Geometry: final body of the model. Coordinates: model frame, mm. Round coordinates to 2 decimals unless told otherwise and drop trailing zeros. Answer in a Markdown table with one row per item.
```python
from build123d import *

# Parameters (mm, degrees)
SKETCH1_R           = 2.25
BOSS_EXTRUDE1_DEPTH = 28


with BuildPart() as part:
    # Sketch1 → Boss-Extrude1 (new body)
    with BuildSketch(Plane(origin=(0, 0, 0), x_dir=(0, 0, -1), z_dir=(1, 0, 0))):
        with BuildLine():
            Line((-150, 25), (150, 25))
            add(Edge.make_bspline(
                [(150, 25), (230, 0), (150, -25)],
                knots=[0, 0, 0, 1, 1, 1], degree=2))
            Line((150, -25), (-150, -25))
            add(Edge.make_bspline(
                [(-150, 25), (-230, 0), (-150, -25)],
                knots=[0, 0, 0, 1, 1, 1], degree=2))
        make_face()
        with Locations((-175, 0)):
            Circle(SKETCH1_R, mode=Mode.SUBTRACT)
        with Locations((175, 0)):
            Circle(SKETCH1_R, mode=Mode.SUBTRACT)
    extrude(amount=BOSS_EXTRUDE1_DEPTH)


solid = part.part
```
Item 1: Ray query, L1, parallel to Y at x = 9.25, z = 175; L2, parallel to Y at x = 21, z = 165; L3, parallel to Z at x = 25.75, y = -19.5. Return the intervals inside material, ascending.
Ans:
| item | result |
|---|---|
| L1 | -15.31 to -2.25, 2.25 to 15.31 |
| L2 | -19.76 to 19.76 |
| L3 | -165.66 to 165.66 |
Item 2: First-contact query: P1, Ø7, axis at y = 0, z = 175, coming from the -X side; P2, Ø5, axis at x = 3, y = 19, coming from the +Z side; P3, Ø8, axis at x = 15, y = -15.5, coming from the -Z side; P4, Ø6, axis at x = 23, y = 16, coming from the +Z side. Flat tips, straight axial feed; report the tip coordinate or a pass-through.
Ans:
| item | result |
|---|---|
| P1 | x = 0 |
| P2 | z = 172.58 |
| P3 | z = -181.54 |
| P4 | z = 179.18 |
Item 3: Section query A-A, the plane x = 11.5. State how many separate pieces and enclosed holes the cut face has, and give its area (3 significant figures).
Ans:
| item | result |
|---|---|
| separate pieces | 1 |
| enclosed holes | 2 |
| area | 17,600 mm2 |
